Input: part model. Units: mm. Frame: model coordinates. A direction names the side the tool comes from. Give positions to 0.01 mm unless a question says otherwise; leave off trailing zeros. Loops run counter-clockwise (first coordinate to the right, second up) from the corner with the lowest first, then second, coordinate; pieces in that order, holes last. Notation, with made-up numbers: M 42.5,60.25 L 69.5,60.25 A25 ccw 69.5,76.25 Z; hole C 47,80 d11. An arc over 180 degrees is marked long. One line per item, written item: value. Start each with the question number.
(1) Pin query (flat end, axial travel): P1, Ø5.5, axis at y = 0.5, z = -1, coming from the +X side; P2, Ø3, axis at x = 0, z = 0, coming from the +Y side; P3, Ø3, axis at x = 0, z = 0, coming from the -Y side; P4, Ø3, axis at x = 0, y = 0, coming from the -Z side. Return the tip coordinate at first contact, or that it passes through.
(2) Section B-B on y = 0. Output: boundary loops of the cut face in (x, z) (3 decimals).
(3) Access query for faces 1 (the cylindrical face through (2.307, -4.436, -8.649)), 2 (the cylindrical face through (-0.53, -2.387, 9.042)), 3 (the cylindrical face through (8, 0, -5)), 4 (the flat face through (-6, 0, 0)), 5 (the cylindrical face through (-1.49, -9.04, -1.94)). Directions: +Z, -Z, +X, -X, +Y, -Y. A direction counts if a zero-diameter tool reaches every point of the face in a straight line with its end or side. Return the directions, or none.
(4) Section C-C on x = 9.5. Output: boundary loops of the cut face in (y, z) (3 decimals), plus the area to 3 significant figures.
(5) Section A-A on z = 3. Output: boundary loops of the cut face in (x, y), plus the area to 3 significant figures.
(6) Pull-direction query (Z, two-part tool) for faces 6 (the cylindrical face through (9.042, -2.387, -0.53)), 7 (the flat face through (0, 0, 6)), 8 (the cylindrical face through (-8.649, -4.434, 2.31)); classes: released by +Z, released by -Z, zero draft, split by the parting line, or undercut.
(7) Ray query, line 1 along Y through (x, z) = (0, -10.5) (3 decimals); line 2 along Z through (x, y) = (8, -0.25). Return the intervals inside material, ascending. Write a range as from..to.
```python
from build123d import *

# Parameters (mm, degrees)
IZIM1_R                     = 5
Y_KSEKLIK_EKSTR_ZYON1_DEPTH = 12
IZIM2_R                     = 5
Y_KSEKLIK_EKSTR_ZYON2_DEPTH = 12
IZIM3_R                     = 5
Y_KSEKLIK_EKSTR_ZYON3_DEPTH = 12
IZIM4_R                     = 2.445
KES_EKSTR_ZYON1_DEPTH       = 6
IZIM5_R                     = 2.445
KES_EKSTR_ZYON2_DEPTH       = 6
IZIM6_R                     = 2.445
KES_EKSTR_ZYON3_DEPTH       = 6


with BuildPart() as part:
    # Çizim1 → Yükseklik-Ekstrüzyon1 (new, symmetric)
    with BuildSketch(Plane.XY):
        Circle(IZIM1_R)
    extrude(amount=Y_KSEKLIK_EKSTR_ZYON1_DEPTH, both=True)

    # Çizim2 → Yükseklik-Ekstrüzyon2 (add, symmetric)
    with BuildSketch(Plane(origin=(0, 0, 0), x_dir=(1, 0, 0), z_dir=(0, 1, 0))):
        Circle(IZIM2_R)
    extrude(amount=Y_KSEKLIK_EKSTR_ZYON2_DEPTH, both=True)

    # Çizim3 → Yükseklik-Ekstrüzyon3 (add, symmetric)
    with BuildSketch(Plane(origin=(0, 0, 0), x_dir=(0, 0, -1), z_dir=(1, 0, 0))):
        with Locations(Location((0, 0, 0), (0, 0, 225))):
            Circle(IZIM3_R)
    extrude(amount=Y_KSEKLIK_EKSTR_ZYON3_DEPTH, both=True)

    # Çizim4 → Kes-Ekstrüzyon1 (cut)
    with BuildSketch(Plane.ZY.offset(12)):
        Circle(IZIM4_R)
    kes_ekstr_zyon1 = extrude(amount=-KES_EKSTR_ZYON1_DEPTH, mode=Mode.SUBTRACT)

    # Aynalama1: Kes-Ekstrüzyon1 across plane
    add(kes_ekstr_zyon1.mirror(Plane(origin=(0, 0, 0), x_dir=(0, 0, 1), z_dir=(1, 0, 0))), mode=Mode.SUBTRACT)

    # Çizim5 → Kes-Ekstrüzyon2 (cut)
    with BuildSketch(Plane.XY.offset(12)):
        Circle(IZIM5_R)
    kes_ekstr_zyon2 = extrude(amount=-KES_EKSTR_ZYON2_DEPTH, mode=Mode.SUBTRACT)

    # Aynalama2: Kes-Ekstrüzyon2 across plane
    add(kes_ekstr_zyon2.mirror(Plane.XY), mode=Mode.SUBTRACT)

    # Çizim6 → Kes-Ekstrüzyon3 (cut)
    with BuildSketch(Plane(origin=(0, 12, 0), x_dir=(1, 0, 0), z_dir=(0, 1, 0))):
        with Locations(Location((0, 0, 0), (0, 0, 270))):
            Circle(IZIM6_R)
    kes_ekstr_zyon3 = extrude(amount=-KES_EKSTR_ZYON3_DEPTH, mode=Mode.SUBTRACT)

    # Aynalama3: Kes-Ekstrüzyon3 across plane
    add(kes_ekstr_zyon3.mirror(Plane.ZX), mode=Mode.SUBTRACT)


solid = part.part
```
Output values:
1. P1: stops at x = 12
1. P2: stops at y = 6
1. P3: stops at y = -6
1. P4: stops at z = -6
2. outline: M -12,-5 L -5,-5 L -5,-12 L -2.445,-12 L -2.445,-6 L 2.445,-6 L 2.445,-12 L 5,-12 L 5,-5 L 12,-5 L 12,-2.445 L 6,-2.445 L 6,2.445 L 12,2.445 L 12,5 L 5,5 L 5,12 L 2.445,12 L 2.445,6 L -2.445,6 L -2.445,12 L -5,12 L -5,5 L -12,5 L -12,2.445 L -6,2.445 L -6,-2.445 L -12,-2.445 Z
3. face 1: -Z
3. face 2: +Z
3. face 3: +X
3. face 4: -X
3. face 5: -Y
4. outline: C 0,0 d10; hole C 0,0 d4.89
4. area: 59.8 mm²
5. outline: M -12,-4 L -4,-4 L -4,-12 L 4,-12 L 4,-4 L 12,-4 L 12,4 L 4,4 L 4,12 L -4,12 L -4,4 L -12,4 Z
5. area: 320 mm²
6. face 6: undercut
6. face 7: released by +Z
6. face 8: split by the parting line
7. line 1: y = -5..-2.445, 2.445..5
7. line 2: z = -4.99..-2.43, 2.43..4.99
